Work out the finished part from the listing and answer in its coordinate system (mm). Give positions to 0.01 mm unless a question says otherwise; leave off trailing zeros. Loops run counter-clockwise (first coordinate to the right, second up) from the corner with the lowest first, then second, coordinate; pieces in that order, holes last. Notation, with made-up numbers: M 31,-18 L 62,-18 A21 cw 62,-14 Z; hole C 38,36.5 d7. An arc over 180 degrees is marked long. Write item = value, one per line. Start each with the question number.
1. Flat-ended cylindrical pins translate along their axes: pin 1 Ø1.8 at (x, z) = (-121.62, -77.85) entering from +Y; pin 2 Ø1.2 at (x, y) = (32, 2) entering from +Z. Find the tip coordinate at first contact, or state that the pin passes through.
2. Section A-A on z = 66 is taken. Determine the outline of the cut face in (x, y), plus the area to 3 significant figures.
3. Section B-B on x = 42.5 is taken. Determine the outline of the cut face in (y, z).
4. Section D-D on y = 0.65 is taken. Give the number of separate pieces and of enclosed holes in the cut face, plus the area to 3 significant figures.
5. Consider L1, parallel to X at y = 1.7, z = 28.85; L2, parallel to Z at x = -29.5, y = 3.5; L3, parallel to X at y = 1.65, z = -36. Determine where each line is inside the solid, lowest interval first. Write a range as [from, to].
6. Section C-C on z = 105 is taken. Determine the outline of the cut face in (x, y), plus the area to 3 significant figures.
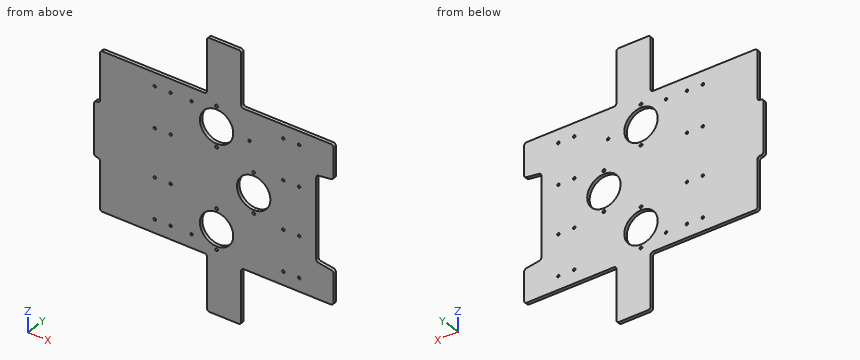
```python
from build123d import *

# Parameters (mm, degrees)
SKETCH1_R           = 20
SKETCH1_R_2         = 1.5
SKETCH1_R_3         = 1.65
BOSS_EXTRUDE2_DEPTH = 4
FILLET1_R           = 3


with BuildPart() as part:
    # Sketch1 → Boss-Extrude2 (new body)
    with BuildSketch(Plane(origin=(0, 0, 0), x_dir=(1, 0, 0), z_dir=(0, 1, 0))):
        Polygon((92.45867298, 93.85), (92.45867298, 53.803836873), (71.914755495, 50.55), (71.914755495, -50.55), (92.528223413, -53.3293777), (92.45867298, -93.85), (-18.04132702, -93.85), (-18.04132702, -160.15), (-59.04132702, -160.15), (-59.04132702, -93.85), (-187.29132702, -93.85), (-187.29132702, -32.5), (-194.29132702, -32.5), (-194.29132702, 32.5), (-187.29132702, 32.5), (-187.29132702, 34.274594508), (-187.29132702, 93.85), (-59.04132702, 93.85), (-59.04132702, 160.15), (-18.04132702, 160.15), (-18.04132702, 93.85), align=None)
        with Locations(Location((-47.54132702, 60, 0), (0, 0, 270))):
            Circle(SKETCH1_R, mode=Mode.SUBTRACT)
        with Locations(Location((-3.085244505, 0, 0), (0, 0, 270))):
            Circle(SKETCH1_R, mode=Mode.SUBTRACT)
        with Locations(Location((-47.54132702, -60, 0), (0, 0, 90))):
            Circle(SKETCH1_R, mode=Mode.SUBTRACT)
        with Locations(Location((-77.54132702, 77.85, 0), (0, 0, 270))):
            Circle(SKETCH1_R_2, mode=Mode.SUBTRACT)
        with Locations(Location((-121.62132702, 28.85, 0), (0, 0, 270))):
            Circle(SKETCH1_R_2, mode=Mode.SUBTRACT)
        with Locations(Location((-102.65132702, 28.85, 0), (0, 0, 270))):
            Circle(SKETCH1_R_2, mode=Mode.SUBTRACT)
        with Locations(Location((-121.62132702, -28.85, 0), (0, 0, 90))):
            Circle(SKETCH1_R_2, mode=Mode.SUBTRACT)
        with Locations(Location((-102.65132702, -28.85, 0), (0, 0, 90))):
            Circle(SKETCH1_R_2, mode=Mode.SUBTRACT)
        with Locations(Location((-77.54132702, -77.85, 0), (0, 0, 90))):
            Circle(SKETCH1_R_2, mode=Mode.SUBTRACT)
        with Locations(Location((32.45867298, 77.85, 0), (0, 0, 270))):
            Circle(SKETCH1_R_2, mode=Mode.SUBTRACT)
        with Locations(Location((-8.085244505, -58.85, 0), (0, 0, 270))):
            Circle(SKETCH1_R_2, mode=Mode.SUBTRACT)
        with Locations(Location((32.45867298, -77.85, 0), (0, 0, 90))):
            Circle(SKETCH1_R_2, mode=Mode.SUBTRACT)
        with Locations(Location((-121.62132702, -77.85, 0), (0, 0, 90))):
            Circle(SKETCH1_R_2, mode=Mode.SUBTRACT)
        with Locations(Location((-102.65132702, -77.85, 0), (0, 0, 90))):
            Circle(SKETCH1_R_2, mode=Mode.SUBTRACT)
        with Locations(Location((51.42867298, -77.85, 0), (0, 0, 90))):
            Circle(SKETCH1_R_2, mode=Mode.SUBTRACT)
        with Locations(Location((32.444755495, -28.85, 0), (0, 0, 90))):
            Circle(SKETCH1_R_2, mode=Mode.SUBTRACT)
        with Locations(Location((51.414755495, -28.85, 0), (0, 0, 90))):
            Circle(SKETCH1_R_2, mode=Mode.SUBTRACT)
        with Locations(Location((-121.62132702, 77.85, 0), (0, 0, 270))):
            Circle(SKETCH1_R_2, mode=Mode.SUBTRACT)
        with Locations(Location((-102.65132702, 77.85, 0), (0, 0, 270))):
            Circle(SKETCH1_R_2, mode=Mode.SUBTRACT)
        with Locations(Location((51.414755495, 28.85, 0), (0, 0, 270))):
            Circle(SKETCH1_R_2, mode=Mode.SUBTRACT)
        with Locations(Location((32.444755495, 28.85, 0), (0, 0, 270))):
            Circle(SKETCH1_R_2, mode=Mode.SUBTRACT)
        with Locations(Location((51.42867298, 77.85, 0), (0, 0, 270))):
            Circle(SKETCH1_R_2, mode=Mode.SUBTRACT)
        with Locations(Location((-47.54132702, -84, 0), (0, 0, 270))):
            Circle(SKETCH1_R_3, mode=Mode.SUBTRACT)
        with Locations(Location((-47.54132702, -36, 0), (0, 0, 270))):
            Circle(SKETCH1_R_3, mode=Mode.SUBTRACT)
        with Locations(Location((-3.085244505, -24, 0), (0, 0, 270))):
            Circle(SKETCH1_R_3, mode=Mode.SUBTRACT)
        with Locations(Location((-3.085244505, 24, 0), (0, 0, 270))):
            Circle(SKETCH1_R_3, mode=Mode.SUBTRACT)
        with Locations(Location((-47.54132702, 36, 0), (0, 0, 270))):
            Circle(SKETCH1_R_3, mode=Mode.SUBTRACT)
        with Locations(Location((-47.54132702, 84, 0), (0, 0, 270))):
            Circle(SKETCH1_R_3, mode=Mode.SUBTRACT)
    extrude(amount=BOSS_EXTRUDE2_DEPTH)

    # Fillet1
    fillet1_edges = [part.edges().sort_by_distance(p)[0] for p in [
        (-187.29132702, 2, -93.85),
        (-59.04132702, 2, -93.85),
        (-59.04132702, 2, -160.15),
        (-18.04132702, 2, -160.15),
        (-18.04132702, 2, -93.85),
        (92.45867298, 2, -93.85),
        (92.45867298, 2, -53.803836873),
        (71.914755495, 2, -50.55),
        (71.914755495, 2, 50.55),
        (92.528223413, 2, 53.3293777),
        (92.45867298, 2, 93.85),
        (-18.04132702, 2, 93.85),
        (-18.04132702, 2, 160.15),
        (-59.04132702, 2, 160.15),
        (-59.04132702, 2, 93.85),
        (-187.29132702, 2, 93.85),
        (-187.29132702, 2, 32.5),
        (-194.29132702, 2, 32.5),
        (-194.29132702, 2, -32.5),
        (-187.29132702, 2, -32.5),
    ]]
    fillet(fillet1_edges, radius=FILLET1_R)


solid = part.part
```
Verdict:
q1.pin_1 = through
q1.pin_2 = 93.85
q2.outline = M -187.29,0 L -66.62,0 L -66.62,4 L -187.29,4 Z; M -28.46,0 L 92.51,0 L 92.51,4 L -28.46,4 Z
q2.area = 967 mm2
q3.outline = M 0,-93.85 L 4,-93.85 L 4,93.85 L 0,93.85 Z
q4.separate_pieces = 1
q4.enclosed_holes = 28
q4.area = 52,300 mm2
q5.L1 = [-194.29, -123.12], [-120.12, -104.15], [-101.15, 30.94], [33.94, 49.91], [52.91, 71.91]
q5.L2 = [-160.15, -68.63], [-51.37, 51.37], [68.63, 160.15]
q5.L3 = [-187.29, -49.19], [-45.89, 71.91]
q6.outline = M -59.04,0 L -18.04,0 L -18.04,4 L -59.04,4 Z
q6.area = 164 mm2
